Design review of the part built by this model. Coordinates are the model's own, in mm. A direction names the side the tool comes from. Coordinates: 2 decimals unless noted, no trailing zeros. Write each loop counter-clockwise with the first axis right and the second up, starting at its lowest first coordinate (ties: lowest second). Pieces come first, ordered by that corner, then holes. Notation, with made-up numbers: M -23,30.5 L -16,30.5 A22 ccw -16,44.5 Z; hole C 48,-22 d1. An arc over 180 degrees is marked long. Return JSON: item names as keys, results as strings. Group by question number.
```python
from build123d import *

# Parameters (mm, degrees)
EXTRUDE_1_DEPTH          = 10
SKETCH_2_R               = 335.5
EXTRUDE_2_DEPTH          = 206
EXTRUDE_3_REACH          = 639.278
SHELL_1_T                = -5
SKETCH_4_R               = 80
EXTRUDE_4_DEPTH          = 61.8
EXTRUDE_START            = 128.6
SKETCH_5_R               = 80
EXTRUDE_5_DEPTH          = 128.6
SKETCH_7_R               = 48
CUT_EXTRUDE_1_DEPTH      = 661.787443131
RIB_START                = -5
RIB_2_DEPTH              = 10
PATTERN_CIRCULAR_2_COUNT = 6
RIB_9_REACH              = 662.787
SKETCH_13_WALL_W         = 1624.932905634
SKETCH_13_WALL_H         = 10
FILLET_1_R               = 10
FILLET_2_R               = 10
FILLET_3_R               = 10


# Read off the part's stored shape, not the designer's step: 筋2
with BuildPart() as part:
    # 草图1 → 凸台-拉伸1 (new body)
    with BuildSketch(Plane(origin=(0, 0, 0), x_dir=(1, 0, 0), z_dir=(0, 1, 0))):
        with BuildLine():
            ThreePointArc((145.890781066, -423.95), (171.576116901, -414.221388401), (196.61755928, -402.938280488))
            Line((196.61755928, -402.938280488), (402.938280488, -196.61755928))
            ThreePointArc((402.938280488, -196.61755928), (414.221388401, -171.576116901), (423.95, -145.890781066))
            Line((423.95, -145.890781066), (423.95, 145.890781066))
            ThreePointArc((423.95, 145.890781066), (414.221388401, 171.576116901), (402.938280488, 196.61755928))
            Line((402.938280488, 196.61755928), (196.61755928, 402.938280488))
            ThreePointArc((196.61755928, 402.938280488), (171.576116901, 414.221388401), (145.890781066, 423.95))
            Line((145.890781066, 423.95), (-145.890781066, 423.95))
            ThreePointArc((-145.890781066, 423.95), (-171.576116901, 414.221388401), (-196.61755928, 402.938280488))
            Line((-196.61755928, 402.938280488), (-402.938280488, 196.61755928))
            ThreePointArc((-402.938280488, 196.61755928), (-414.221388401, 171.576116901), (-423.95, 145.890781066))
            Line((-423.95, 145.890781066), (-423.95, -145.890781066))
            ThreePointArc((-423.95, -145.890781066), (-414.221388401, -171.576116901), (-402.938280488, -196.61755928))
            Line((-402.938280488, -196.61755928), (-196.61755928, -402.938280488))
            ThreePointArc((-196.61755928, -402.938280488), (-171.576116901, -414.221388401), (-145.890781066, -423.95))
            Line((-145.890781066, -423.95), (145.890781066, -423.95))
        make_face()
    extrude(amount=EXTRUDE_1_DEPTH)

    # 草图2 → 凸台-拉伸2 (add)
    with BuildSketch(Plane(origin=(0, 10, 0), x_dir=(1, 0, 0), z_dir=(0, 1, 0))):
        with Locations(Location((0, 0, 0), (0, 0, 270))):
            Circle(SKETCH_2_R)
    extrude(amount=EXTRUDE_2_DEPTH)

    # 草图3 → 凸台-拉伸3 (add, up to next)
    with BuildSketch(Plane(origin=(0, 216, 0), x_dir=(1, 0, 0), z_dir=(0, 1, 0)), mode=Mode.PRIVATE) as extrude_3_sk1:
        with BuildLine():
            ThreePointArc((298.83774862, 152.5), (326.205697882, 78.422526541), (335.5, 0))
            Line((335.5, 0), (374.873930941, 0))
            Line((374.873930941, 0), (374.873930941, 152.5))
            Line((374.873930941, 152.5), (298.83774862, 152.5))
        make_face()
    extrude_3_tool1 = extrude(extrude_3_sk1.sketch, amount=-EXTRUDE_3_REACH, mode=Mode.PRIVATE) - part.part
    # 草图3 → 凸台-拉伸3 (add, up to next)
    with BuildSketch(Plane(origin=(0, 216, 0), x_dir=(1, 0, 0), z_dir=(0, 1, 0)), mode=Mode.PRIVATE) as extrude_3_sk2:
        with BuildLine():
            Line((374.873930941, 0), (335.5, 0))
            ThreePointArc((335.5, 0), (326.205697882, -78.422526541), (298.83774862, -152.5))
            Line((298.83774862, -152.5), (374.873930941, -152.5))
            Line((374.873930941, -152.5), (374.873930941, 0))
        make_face()
    extrude_3_tool2 = extrude(extrude_3_sk2.sketch, amount=-EXTRUDE_3_REACH, mode=Mode.PRIVATE) - part.part
    add(extrude_3_tool1.solids().sort_by_distance((348.072526, 216, -85.221274))[0])
    add(extrude_3_tool2.solids().sort_by_distance((348.072526, 216, 85.221274))[0])

    # 抽壳1
    shell_1_openings = [part.faces().sort_by_distance(p)[0] for p in [
        (0, 0, 0),
    ]]
    offset(amount=SHELL_1_T, openings=shell_1_openings, kind=Kind.INTERSECTION)

    # 草图4 → 凸台-拉伸4 (add)
    with BuildSketch(Plane(origin=(0, 216, 0), x_dir=(1, 0, 0), z_dir=(0, 1, 0))):
        with Locations(Location((0, 0, 0), (0, 0, 90))):
            Circle(SKETCH_4_R)
    extrude(amount=EXTRUDE_4_DEPTH)

    # 草图5 → 凸台-拉伸5 (add)
    with BuildSketch(Plane.XZ.offset(-211).offset(EXTRUDE_START)):
        with Locations(Location((0, 0, 0), (0, 0, 270))):
            Circle(SKETCH_5_R)
    extrude(amount=-EXTRUDE_5_DEPTH)

    # 草图7 → 切除-拉伸1 (cut, through all)
    with BuildSketch(Plane(origin=(0, 277.8, 0), x_dir=(1, 0, 0), z_dir=(0, 1, 0))):
        with Locations(Location((0, 0, 0), (0, 0, 270))):
            Circle(SKETCH_7_R)
    extrude(amount=-CUT_EXTRUDE_1_DEPTH, mode=Mode.SUBTRACT)

    # 筋2 outline → 筋2 (add)
    with BuildSketch(Plane.XY.offset(RIB_START)):
        Polygon((-330.5, 109.315910213), (-79.843597113, 87.38631652), (-78, 87.225022673), (-78, 211), (-332, 211), (-332, 109.447143208), align=None)
    rib_2 = extrude(amount=RIB_2_DEPTH)

    # 阵列(圆周)2: 筋2 ×6 about axis, 1 skipped
    pattern_circular_2_axis = Axis((0, 0, 0), (0, 1, 0))
    add([rib_2.rotate(pattern_circular_2_axis, i * 360 / PATTERN_CIRCULAR_2_COUNT) for i in range(1, PATTERN_CIRCULAR_2_COUNT) if i not in (3,)])

    # 草图13 wall → 筋9 (add, up to next)
    with BuildSketch(Plane(origin=(224.936965471, 128.6, 0), x_dir=(0.961892208962, 0.2734289274, 0), z_dir=(-0.2734289274, 0.961892208962, 0)), mode=Mode.PRIVATE) as rib_9_sk1:
        Rectangle(SKETCH_13_WALL_W, SKETCH_13_WALL_H)
    rib_9_tool1 = extrude(rib_9_sk1.sketch, amount=RIB_9_REACH, mode=Mode.PRIVATE) - part.part
    add(rib_9_tool1.solids().sort_by_distance((224.936965471, 128.6, 0))[0])

    # 圆角1
    fillet_1_edges = [part.edges().sort_by_distance(p)[0] for p in [
        (374.873930941, 113, -152.5),
        (336.85583978, 216, -152.5),
    ]]
    fillet(fillet_1_edges, radius=FILLET_1_R)

    # 圆角2
    # the kernel refuses this fillet: 10 mm, written as the material it adds along each edge
    with BuildSketch(Plane(origin=(369.873930941, 211, -5), x_dir=(-1, 0, 0), z_dir=(0, 0, -1))) as fillet_2_piece_1:
        with BuildLine():
            CenterArc((FILLET_2_R, -FILLET_2_R), FILLET_2_R, 90, 90)
            Line((0, -FILLET_2_R), (0, 0))
            Line((0, 0), (FILLET_2_R, 0))
        make_face()
    extrude(amount=142.5)
    # the kernel refuses this fillet: 10 mm, written as the material it takes off along each edge
    with BuildSketch(Plane(origin=(364.873930941, 206, -142.5), x_dir=(0, 1, 0), z_dir=(1, 0, 0))) as fillet_2_2_piece_1_section:
        Polygon((0, 0), (FILLET_2_R * 1.02, 0), (FILLET_2_R * 1.02, -FILLET_2_R * 1.02), (0, -FILLET_2_R * 1.02), align=None)
    fillet_2_2_piece_1 = extrude(amount=FILLET_2_R * 1.02, mode=Mode.PRIVATE)
    fillet_2_2_piece_1 = fillet_2_2_piece_1 - Plane(origin=(364.873930941, 206, -142.5), x_dir=(0, -0.7071067811865475, 0.7071067811865475), z_dir=(1, 0, 0)) * Sphere(FILLET_2_R, mode=Mode.PRIVATE)
    add(fillet_2_2_piece_1, mode=Mode.SUBTRACT)
    with BuildSketch(Plane(origin=(374.873930941, 216, -142.5), x_dir=(0, -1, 0), z_dir=(0, 0, 1))) as fillet_2_2_piece_2:
        with BuildLine():
            CenterArc((FILLET_2_R, -FILLET_2_R), FILLET_2_R, 90, 90)
            Line((0, -FILLET_2_R), (0, 0))
            Line((0, 0), (FILLET_2_R, 0))
        make_face()
    extrude(amount=320, mode=Mode.SUBTRACT)

    # 圆角3
    fillet_3_edges = [part.edges().sort_by_distance(p)[0] for p in [
        (331.85583978, 216, 152.5),
        (371.944998753, 213.071067812, 152.5),
        (374.873930941, 108, 152.5),
    ]]
    fillet(fillet_3_edges, radius=FILLET_3_R)


solid = part.part
```
Item 1: Add section B-B (y = 241). Write out the cut boundary in (x, z), plus the area to 3 significant figures.
Item 2: For line 1 (X direction, y = 100.5, z = -17); line 2 (X direction, y = 230, z = 0); line 3 (Z direction, x = -88, y = 166), list the stretches that pass through material, from the lowest coordinate up.
Item 3: Add section C-C (z = 233). Write out the cut boundary in (x, y), plus the area to 3 significant figures.
Item 4: Add section D-D (x = -119.5). Write out the cut boundary in (y, z).
Item 5: The part is to be moulded in two halves that separate along Z. For faces 1 (the cylindrical face through (-171.931, 4.93, 414.074)), 2 (the flat face through (332, 109, 147.5)), 3 (the flat face through (88, 216, -5)), 4 (the cylindrical face through (171.931, 4.93, -414.074)), say which applies: pulls with the +Z half, pulls with the -Z half, needs draft (parallel to the pull), parting line crosses it, or undercut.
Item 6: Add section A-A (x = 0). Write out the cut boundary in (y, z), plus the area to 3 significant figures.
Item 7: Machinability: for faces 5 (the flat face through (-99.123, 150.058, -181.687)), 6 (the cylindrical face through (414.37, 4.93, -171.22)), which of the approach directions +Z, -Z, +X, -X, +Y, -Y give a long, thin tool a straight path to every point of the face, cutting with its end or side? Answer none if there is none.
Item 8: For pin 1 (6 mm diameter, centred on x = -192.5, z = -271.5, fed in from +Y); pin 2 (3 mm diameter, centred on x = 158.5, y = 81, fed in from +Z); pin 3 (5 mm diameter, centred on x = 269, y = 29, fed in from +Z), all flat-tipped, find the tip position at first contact; note any pin that passes through.
Geometry check:
{
 "1": {"outline": "C 0,0 d160; hole C 0,0 d96", "area": "12,900 mm^2"},
 "2": {"line 1": "-335.07 to -330.06, -78.17 to -44.89, 44.89 to 78.17, 369.87 to 374.87", "line 2": "-80 to -48, 48 to 80", "line 3": "-323.75 to -318.57, -162.42 to -142.42, -5 to 5, 142.42 to 162.42, 318.57 to 323.75"},
 "3": {"outline": "M -366.56,0 L -359.48,0 L -359.48,5 L -234.4,5 L -234.4,211 L -140.3,211 L -140.3,104.19 L -128.75,103.69 L -128.75,211 L 128.75,211 L 128.75,103.69 L 140.3,104.19 L 140.3,211 L 234.4,211 L 234.4,5 L 359.48,5 L 359.48,0 L 366.56,0 L 366.56,10 L 241.39,10 L 241.39,216 L -241.39,216 L -241.39,10 L -366.56,10 Z", "area": "9,090 mm^2"},
 "4": {"outline": "M 0,-423.95 L 10,-423.95 L 10,-313.5 L 216,-313.5 L 216,313.5 L 10,313.5 L 10,423.95 L 0,423.95 L 0,418.95 L 5,418.95 L 5,308.14 L 211,308.14 L 211,216.98 L 102.07,216.98 L 100.55,196.98 L 211,196.98 L 211,5 L 90.86,5 L 90.86,-5 L 211,-5 L 211,-196.98 L 100.55,-196.98 L 102.07,-216.98 L 211,-216.98 L 211,-308.14 L 5,-308.14 L 5,-418.95 L 0,-418.95 Z"},
 "5": {"face 1": "pulls with the +Z half", "face 2": "undercut", "face 3": "needs draft", "face 4": "pulls with the -Z half"},
 "6": {"outline": "M 0,-423.95 L 10,-423.95 L 10,-335.5 L 216,-335.5 L 216,-80 L 277.8,-80 L 277.8,-48 L 82.4,-48 L 82.4,-80 L 211,-80 L 211,-330.5 L 5,-330.5 L 5,-418.95 L 0,-418.95 Z; M 0,418.95 L 5,418.95 L 5,330.5 L 211,330.5 L 211,80 L 82.4,80 L 82.4,48 L 277.8,48 L 277.8,80 L 216,80 L 216,335.5 L 10,335.5 L 10,423.95 L 0,423.95 Z", "area": "18,100 mm^2"},
 "7": {"face 5": "-Y", "face 6": "-Z, +X, +Y, -Y"},
 "8": {"pin 1": "y = 216", "pin 2": "z = 296.5", "pin 3": "z = 203.81"}
}
